Answer from the drawing. Dimensions are ordinates in mm from the lowest x, y and z of the part. Give positions to 0.01 mm unless a question says otherwise; leave off trailing zeros. Order: outer loops, then holes, each group sorted by start corner. A loop starts at its lowest first (then second) coordinate and runs counter-clockwise, first axis right, second up. Notation, with made-up numbers: (18.5, -30.5) - (54.5, -30.5) arc R17 ccw to (54.5, 2.5) - close; hole circle Ø9 at (36.5, -17). An arc over 180 degrees is marked (long way). Write each question's results on one line, items separated by ' | '.
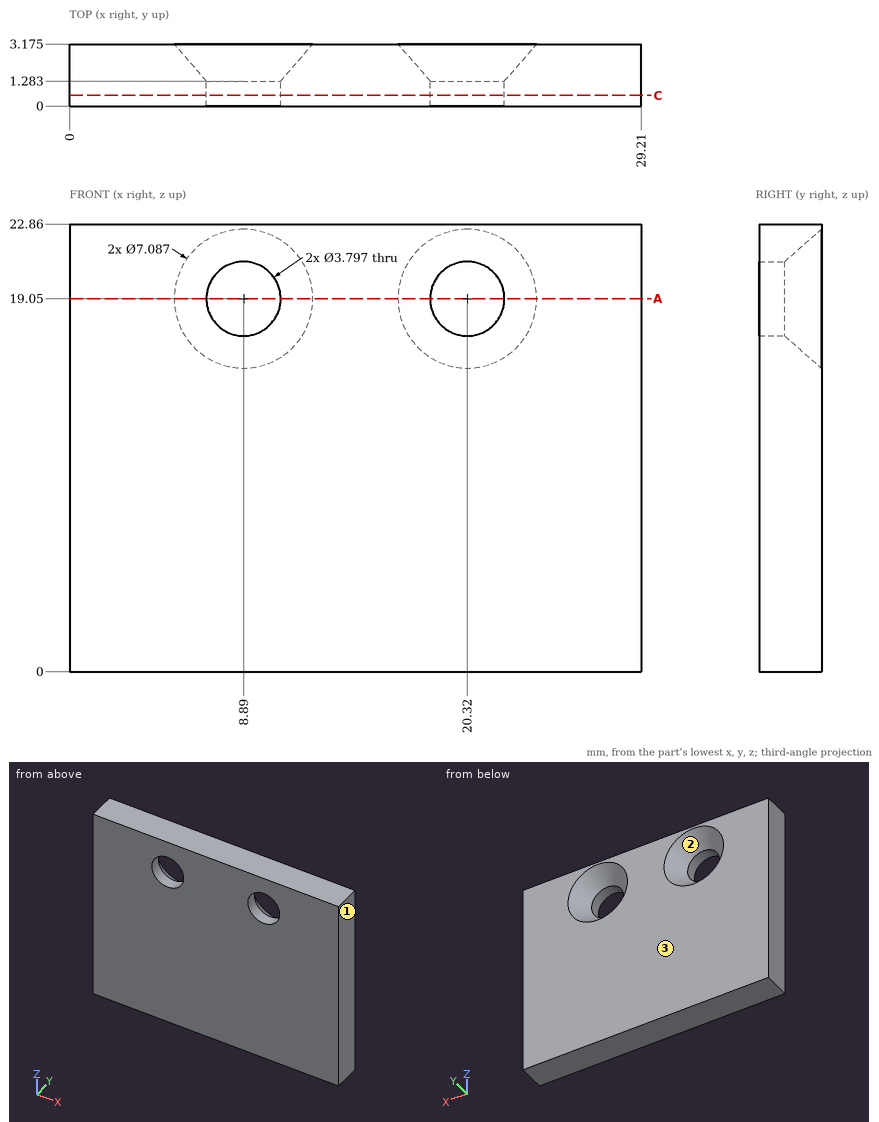
1. Determine the mould class of the marked faces 1, 2 and 3 for opening direction X: +X half, -X half, draft (parallel to the pull), parting line (faces both ways), or undercut.
Answer list:
face 1: +X half | face 2: undercut | face 3: draft
2. A cutting plane is placed at C-C, the plane y = 0.55. Write down the section's boundary in (x, z).
Answer list:
outline: (0, 0) - (29.21, 0) - (29.21, 22.86) - (0, 22.86) - close; hole circle Ø3.8 at (8.89, 19.05); hole circle Ø3.8 at (20.32, 19.05)
3. A cutting plane is placed at A-A, the plane z = 19.05. Write down the section's boundary in (x, y) (1 decimal).
Answer list:
outline: (0, 0) - (7, 0) - (7, 1.3) - (5.3, 3.2) - (0, 3.2) - close; (10.8, 0) - (18.4, 0) - (18.4, 1.3) - (16.8, 3.2) - (12.4, 3.2) - (10.8, 1.3) - close; (22.2, 0) - (29.2, 0) - (29.2, 3.2) - (23.9, 3.2) - (22.2, 1.3) - close
4. Straight lines are drawn through the part: line 1 (X direction, y = 0.85, z = 19.05); line 2 (Z direction, x = 8.89, y = 0.8); line 3 (X direction, y = 0.9, z = 20.25). For each, find the intervals that lie inside material, in ascending order. Write a range as [from, to].
Answer list:
line 1: [0, 6.99], [10.79, 18.42], [22.22, 29.21] | line 2: [0, 17.15], [20.95, 22.86] | line 3: [0, 7.42], [10.36, 18.85], [21.79, 29.21]
